Autodesk Inventor part; units mm, degrees
ref_plane "工作平面2" through (132.5, 10, 132.5) normal (0.1218693, 0.9925462, 0) x (0, 0, -1)
ref_plane "YZ Plane" through (0, 0, 0) normal (1, 0, 0) x (0, 1, 0)
ref_plane "XZ Plane" through (0, 0, 0) normal (0, 1, 0) x (-1, 0, 0)
sketch "草圖1" plane through (0, 0, 0) normal (0, 1, 0) x (-1, 0, 0)
  line L0 (132.5, 132.5) -> (-132.5, 132.5)
  line L1 (-132.5, 132.5) -> (-132.5, -132.5)
  line L2 (-132.5, -132.5) -> (132.5, -132.5)
  line L3 (132.5, -132.5) -> (132.5, 132.5)
  line L4 (132.5, 132.5) -> (-132.5, -132.5) construction
  line L5 (-132.5, 132.5) -> (132.5, -132.5) construction
  point P0 (0, 0)
  dimension "d0" = 265
  dimension "d1" = 265
extrude "擠出1" add sketch "草圖1" along normal blind 10
sketch "草圖3" plane through (0, 10, 0) normal (0, 1, 0) x (1, 0, 0)
  line L0 (132.5, -132.5) -> (132.5, 132.5)
  line L1 (132.5, 132.5) -> (-132.5, 132.5)
  line L2 (-132.5, 132.5) -> (-132.5, -132.5)
  line L3 (-132.5, -132.5) -> (132.5, -132.5)
  point P0 (0, 0)
extrude "擠出2" add sketch "草圖3" along normal blind 100
sketch "草圖4" plane through (132.5, 0, 132.5) normal (1, 0, 0) x (0, 0, -1)
  line L0 (0, 0) -> (265, 0)
  line L1 (265, 0) -> (265, 110)
  line L2 (0, 110) -> (265, 110)
  line L3 (0, 0) -> (0, 110)
  line L4 (0, 0) -> (0, 110)
  line L5 (0, 10) -> (265, 10)
  point P0 (132.5, 0)
  dimension "d7" = 10
ref_plane "工作平面2" through (132.5, 10, 132.5) normal (0.1218693, 0.9925462, 0) x (0, 0, -1)
split "分割1" plane through (132.5, 10, 132.5) removes the side toward (0.1218693, 0.9925462, 0)
sketch "草圖5" plane through (0, 0, 0) normal (0, -1, 0) x (1, 0, 0)
  line L0 (-102.5, -102.5) -> (102.5, -102.5) construction
  line L1 (102.5, -102.5) -> (102.5, 102.5) construction
  line L2 (102.5, 102.5) -> (-102.5, 102.5) construction
  line L3 (-102.5, 102.5) -> (-102.5, -102.5) construction
  line L4 (-102.5, -102.5) -> (102.5, 102.5) construction
  line L5 (102.5, -102.5) -> (-102.5, 102.5) construction
  point P0 (0, 0)
  dimension "d9" = 205
  dimension "d10" = 205
hole "孔1" at (-102.5, 0, -102.5) at (102.5, 0, -102.5) at (102.5, 0, 102.5) at (-102.5, 0, 102.5) direction (0, 1, 0) diameter 5.5 depth 8
sketch "草圖6" plane through (-102.5, 8, -102.5) normal (0, -1, 0) x (1, 0, 0)
  circle A0 centre (0, 205) radius 2.75
  circle A1 centre (205, 205) radius 2.75
  circle A2 centre (205, 0) radius 2.75
  circle A3 centre (0, 0) radius 2.75
  circle A4 centre (0, 0) radius 2.75
  circle A5 centre (205, 0) radius 2.75
  circle A6 centre (0, 205) radius 2.75
  point P0 (102.5, 102.5)
hole "孔2" at (-102.5, 8, -102.5) at (102.5, 8, -102.5) at (102.5, 8, 102.5) at (-102.5, 8, 102.5) direction (0, 1, 0) diameter 11 end through all
sketch "草圖7" plane through (132.5, 10, 132.5) normal (0.1218693, 0.9925462, 0) x (0.9925462, -0.1218693, 0)
  line L0 (-215.2937, 30) -> (-45.2937, 30)
  line L1 (-45.2937, 30) -> (-45.2937, 235)
  line L2 (-45.2937, 235) -> (-215.2937, 235)
  line L3 (-215.2937, 235) -> (-215.2937, 30)
  line L4 (-215.2937, 30) -> (-45.2937, 235) construction
  line L5 (-45.2937, 30) -> (-215.2937, 235) construction
  point P0 (-130.2937, 132.5)
  dimension "d25" = 170
  dimension "d26" = 205
hole "孔3" at (-81.1889, 36.2377, 102.5) at (87.5439, 15.5199, 102.5) at (87.5439, 15.5199, -102.5) at (-81.1889, 36.2377, -102.5) direction (-0.1218693, -0.9925462, 0) diameter 3.5 depth 13 counterbore diameter 5.8 counterbore depth 8.6
sketch "草圖8" plane through (0, 0, 0) normal (0, -1, 0) x (1, 0, 0)
  line L0 (-90, 77.5) -> (90, 77.5)
  line L1 (90, 77.5) -> (90, -77.5)
  line L2 (90, -77.5) -> (-90, -77.5)
  line L3 (-90, -77.5) -> (-90, 77.5)
  line L4 (-90, 77.5) -> (90, -77.5) construction
  line L5 (90, 77.5) -> (-90, -77.5) construction
  point P0 (0, 0)
  dimension "d34" = 180
  dimension "d35" = 155
extrude "擠出3" cut sketch "草圖8" against normal through all
fillet "圓角1" radius 50 4 edges at (-132.5, 21.269, 132.5) (-132.5, 21.269, -132.5) (132.5, 5, -132.5) (132.5, 5, 132.5)
properties part number "頸部桌面轉接件"
Source: CAD feature listing. Evaluate the final solid. Frame: model axes, mm. A direction names the side the tool comes from. Coordinates: 2 decimals unless noted, no trailing zeros. Order: outer loops, then holes, each group sorted by start corner. A loop starts at its lowest first (then second) coordinate and runs counter-clockwise, first axis right, second up.
Item 1: First-contact query: P1, Ø3.5, axis at x = -102.5, z = 102.5, coming from the -Y side; P2, Ø9, axis at x = 100, z = -104.5, coming from the +Y side; P3, Ø1, axis at x = -97, z = 31, coming from the -Y side; P4, Ø3, axis at y = 29.5, z = 14.5, coming from the +X side. Flat tips, straight axial feed; report the tip coordinate or a pass-through.
Output values:
P1: passes through
P2: stops at y = 14.54
P3: stops at y = 0
P4: stops at x = -90
Item 2: Cut plane D-D (y = 33). Count the separate pieces of the cut face and the enclosed holes in it, plus the area to 3 significant figures.
Output values:
separate pieces: 1
enclosed holes: 4
area: 13,800 mm2
Item 3: Pull-direction query (X, two-part tool) for faces 1 (the face through (104, 8, 105)), 2 (the face through (90.2, 0, 1.9)), 3 (the face through (-118.242, 21.567, 117.464)), 4 (the face through (87.1, 6.91, 104.39)); classes: pulls with the +X half, pulls with the -X half, needs draft (parallel to the pull), parting line crosses it, or undercut.
Output values:
face 1: undercut
face 2: needs draft
face 3: pulls with the -X half
face 4: undercut
Item 4: Cut plane B-B (x = -66). Return loops of the section in (y, z), plus the area to 3 significant figures.
Output values:
outline: (0, -132.5) - (34.37, -132.5) - (34.37, -77.5) - (0, -77.5) - close; (0, 77.5) - (34.37, 77.5) - (34.37, 132.5) - (0, 132.5) - close
area: 3,780 mm2
Item 5: Set-up query: faces 5 (the face through (-17, 14, -132.5)), 6 (the face through (-81.64, 27.63, -100.61)), 7 (the face through (90, 8, 1)), 8 (the face through (97.047, 11.225, -101.784)), 9 (the face through (-132.5, 21, -1)). Return all of +Z, -Z, +X, -X, +Y, -Y with unobstructed straight access to the full face (end or side cutting, diameter ignored); none if empty.
Output values:
face 5: -Z, +X, -X, +Y, -Y
face 6: none
face 7: +Y, -Y
face 8: +Y
face 9: +Z, -Z, -X, +Y, -Y
Item 6: Material intervals for line 1 (Z direction, x = 102.5, y = 3.5); line 2 (Z direction, x = 79.5, y = 13); line 3 (X direction, y = 4.5, z = -8), sorted ascending.
Output values:
line 1: z = -128.33 to -105.25, -99.75 to 99.75, 105.25 to 128.33
line 2: z = -132.5 to -77.5, 77.5 to 132.5
line 3: x = -132.5 to -90, 90 to 132.5
Item 7: Cut plane C-C (y = 19.5). Return loops of the section in (x, z), plus the area to 3 significant figures.
Output values:
outline: (-132.5, -82.5) arc R50 ccw to (-82.5, -132.5) - (55.13, -132.5) - (55.13, -77.5) - (-90, -77.5) - (-90, 77.5) - (55.13, 77.5) - (55.13, 132.5) - (-82.5, 132.5) arc R50 ccw to (-132.5, 82.5) - close; hole circle Ø11 at (-102.5, -102.5); hole circle Ø11 at (-102.5, 102.5)
area: 26,000 mm2
Item 8: Cut plane A-A (z = 4.5). Return loops of the section in (x, y).
Output values:
outline: (-132.5, 0) - (-90, 0) - (-90, 37.32) - (-132.5, 42.54) - close; (90, 0) - (132.5, 0) - (132.5, 10) - (90, 15.22) - close
